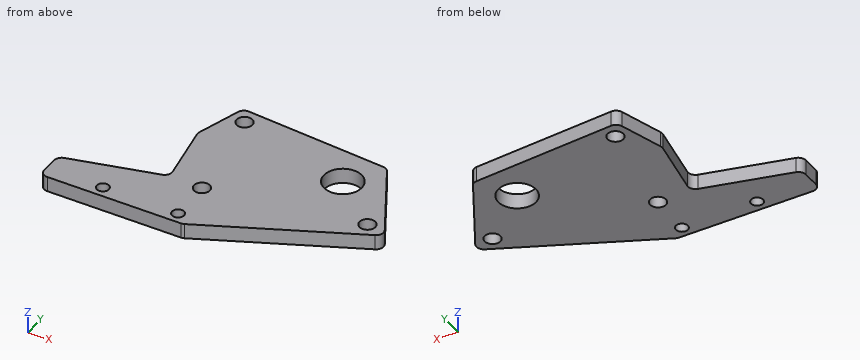
```python
from build123d import *

# Parameters (mm, degrees)
SKETCH1_R           = 2.1
SKETCH1_R_2         = 5
SKETCH1_R_3         = 1.6
BOSS_EXTRUDE1_DEPTH = 4
FILLET1_R           = 2


with BuildPart() as part:
    # Sketch1 → Boss-Extrude1 (new body)
    with BuildSketch(Plane.XY):
        Polygon((0, 0), (-38, 0), (-38, 8), (-12.118525594, 14.647404058), (-15.244192792, 32.373943612), (-11.089131581, 45.719920845), (29.037661116, 42.568648925), (42, 19.629949763), align=None)
        with Locations((-8.219100268, 41.482213208)):
            Circle(SKETCH1_R, mode=Mode.SUBTRACT)
        with Locations((-3.443775383, 14.4)):
            Circle(SKETCH1_R, mode=Mode.SUBTRACT)
        with Locations((36.391698227, 21.424068787)):
            Circle(SKETCH1_R, mode=Mode.SUBTRACT)
        with Locations((22.949568756, 33.015974596)):
            Circle(SKETCH1_R_2, mode=Mode.SUBTRACT)
        with Locations((-23, 3)):
            Circle(SKETCH1_R_3, mode=Mode.SUBTRACT)
        with Locations((-3, 3)):
            Circle(SKETCH1_R_3, mode=Mode.SUBTRACT)
    extrude(amount=BOSS_EXTRUDE1_DEPTH)

    # Fillet1
    fillet1_edges = [part.edges().sort_by_distance(p)[0] for p in [
        (0, 0, 2),
        (-38, 0, 2),
        (-38, 8, 2),
        (-12.118525594, 14.647404058, 2),
        (-15.244192792, 32.373943612, 2),
        (-11.089131581, 45.719920845, 2),
        (29.037661116, 42.568648925, 2),
        (42, 19.629949763, 2),
    ]]
    fillet(fillet1_edges, radius=FILLET1_R)


solid = part.part
```
Read the model definition and answer for the solid it produces. Units are mm, in the model's axes. Give positions to 0.01 mm unless a question says otherwise; leave off trailing zeros. Loops run counter-clockwise (first coordinate to the right, second up) from the corner with the lowest first, then second, coordinate; pieces in that order, holes last.
Item 1: This flat-tipped pin is pushed along its axis until it touches: pin 1 Ø6.5 at (x, y) = (36.39, 21.42) entering from +Z. Where does it stop, or does it pass through?
Item 2: The part is cut by section B-B (x = -3). Write down the section's boundary in (y, z), and give its area (3 significant figures).
Item 3: The part is cut by section A-A (y = 3). Write down the section's boundary in (x, z).
Item 4: The part is cut by section D-D (x = -23). Write down the section's boundary in (y, z).
Item 5: Find the intervals of material crossed by line 1 along Y through (x, z) = (-3, 1.65); line 2 along X through (y, z) = (35, 0.2); line 3 along X through (y, z) = (28.5, 1.8), in increasing order.
Item 6: The part is cut by section C-C (z = 1.4). Write down the section's boundary in (x, y), and give its area (3 significant figures).
Taken from the geometry:
1. pin 1: stops at z = 4
2. outline: (0, 0) - (1.4, 0) - (1.4, 4) - (0, 4) - close; (4.6, 0) - (12.35, 0) - (12.35, 4) - (4.6, 4) - close; (16.45, 0) - (45.08, 0) - (45.08, 4) - (16.45, 4) - close
2. area: 151 mm2
3. outline: (-38, 0) - (-24.6, 0) - (-24.6, 4) - (-38, 4) - close; (-21.4, 0) - (-4.6, 0) - (-4.6, 4) - (-21.4, 4) - close; (-1.4, 0) - (6.42, 0) - (6.42, 4) - (-1.4, 4) - close
4. outline: (0, 0) - (1.4, 0) - (1.4, 4) - (0, 4) - close; (4.6, 0) - (11.85, 0) - (11.85, 4) - (4.6, 4) - close
5. line 1: y = 0 to 1.4, 4.6 to 12.35, 16.45 to 45.08
5. line 2: x = -14.43 to 18.36, 27.54 to 33.31
5. line 3: x = -14.56 to 20.8, 25.1 to 36.99
6. outline: (-38, 2) arc R2 ccw to (-36, 0) - (-0.44, 0) arc R2 ccw to (0.4, 0.19) - (40.04, 18.72) arc R2 ccw to (40.94, 21.51) - (29.56, 41.64) arc R2 ccw to (27.98, 42.65) - (-9.5, 45.59) arc R2 ccw to (-11.56, 44.2) - (-15.1, 32.84) arc R2 ccw to (-15.16, 31.9) - (-12.44, 16.47) arc R2 cw to (-13.91, 14.19) - (-36.5, 8.39) arc R2 ccw to (-38, 6.45) - close; hole circle Ø3.2 at (-23, 3); hole circle Ø4.2 at (-8.22, 41.48); hole circle Ø4.2 at (-3.44, 14.4); hole circle Ø3.2 at (-3, 3); hole circle Ø10 at (22.95, 33.02); hole circle Ø4.2 at (36.39, 21.42)
6. area: 2,010 mm2
